from build123d import *

# Parameters (mm, degrees)
BOSS_EXTRUDE1_DEPTH = 5
SKETCH2_W           = 13.8
SKETCH2_H           = 7
BOSS_EXTRUDE2_DEPTH = 5
SKETCH3_W           = 13.8
SKETCH3_H           = 7
BOSS_EXTRUDE3_DEPTH = 5


with BuildPart() as part:
    # Sketch1 → Boss-Extrude1 (new body)
    with BuildSketch(Plane(origin=(0, 0, 0), x_dir=(1, 0, 0), z_dir=(0, 1, 0))):
        Polygon((132.481495242, 9.8), (132.481495242, 4.8), (142.481495242, 4.8), (152.5, 4.8), (152.5, 0), (142.5, 0), (0, 0), (0, 9.8), align=None)
    extrude(amount=BOSS_EXTRUDE1_DEPTH)

    # Sketch2 → Boss-Extrude2 (add)
    with BuildSketch(Plane.ZY.offset(-10)):
        with Locations((-4.9, 3.5)):
            Rectangle(SKETCH2_W, SKETCH2_H)
    extrude(amount=-BOSS_EXTRUDE2_DEPTH)

    # Sketch3 → Boss-Extrude3 (add)
    with BuildSketch(Plane(origin=(30.2, 0, 0), x_dir=(0, 0, -1), z_dir=(1, 0, 0))):
        with Locations((4.9, 3.5)):
            Rectangle(SKETCH3_W, SKETCH3_H)
    extrude(amount=-BOSS_EXTRUDE3_DEPTH)


solid = part.part
For this review, take the finished solid that the model builds, in its own axes (mm). A direction names the side the tool comes from. Coordinates: 2 decimals unless noted, no trailing zeros. Loops run counter-clockwise (first coordinate to the right, second up) from the corner with the lowest first, then second, coordinate; pieces in that order, holes last. Notation, with made-up numbers: (4, 45.25) -> (37, 45.25) arc R21 ccw to (37, 52.25) -> close; hole circle Ø2 at (-37, 55). An arc over 180 degrees is marked (long way). Write each question's results on one line, items separated by ' | '.
Q1. For pin 1 Ø4 at (x, y) = (138, 2) entering from -Z; pin 2 Ø5 at (x, z) = (6.5, -6.5) entering from +Y; pin 3 Ø2.5 at (x, y) = (82.5, 3) entering from -Z, all flat-tipped, find the tip position at first contact; note any pin that passes through.
Taken from the geometry:
pin 1: z = -4.8 | pin 2: y = 5 | pin 3: z = -9.8
Q2. Add section B-B, the plane y = 3.25. State the section outline as (x, z) points, then the cut area to 3 significant figures.
Taken from the geometry:
outline: (0, -9.8) -> (10, -9.8) -> (10, -11.8) -> (15, -11.8) -> (15, -9.8) -> (25.2, -9.8) -> (25.2, -11.8) -> (30.2, -11.8) -> (30.2, -9.8) -> (132.48, -9.8) -> (132.48, -4.8) -> (152.5, -4.8) -> (152.5, 0) -> (30.2, 0) -> (30.2, 2) -> (25.2, 2) -> (25.2, 0) -> (15, 0) -> (15, 2) -> (10, 2) -> (10, 0) -> (0, 0) -> close | area: 1,430 mm²
Q3. Mouldability with a two-part tool opening along X and no side actions: class faces 4 (the flat face through (152.5, 2, -2)), 5 (the flat face through (15, 6, -5)), 6 (the flat face through (12, 3, 2)) as +X half, -X half, draft (parallel to the pull), parting line (faces both ways), or undercut.
Taken from the geometry:
face 4: +X half | face 5: undercut | face 6: draft
Q4. To check wall thickness, follow line 1 along X through (y, z) = (6.75, -6.75); line 2 along Y through (x, z) = (9, -7.25); line 3 along X through (y, z) = (0.75, -6). State the ranges of each line that lie inside material, in increasing order. Write a range as [from, to].
Taken from the geometry:
line 1: [10, 15], [25.2, 30.2] | line 2: [0, 5] | line 3: [0, 132.48]
Q5. Add section A-A, the plane z = -8.5. State the section outline as (x, y) points, then the cut area to 3 significant figures.
Taken from the geometry:
outline: (0, 0) -> (132.48, 0) -> (132.48, 5) -> (30.2, 5) -> (30.2, 7) -> (25.2, 7) -> (25.2, 5) -> (15, 5) -> (15, 7) -> (10, 7) -> (10, 5) -> (0, 5) -> close | area: 682 mm²
Q6. Machinability: for faces 1 (the flat face through (90, 2, 0)), 2 (the flat face through (20, 5, -5)), 3 (the flat face through (5, 2, 0)), which of the approach directions +Z, -Z, +X, -X, +Y, -Y give a long, thin tool a straight path to every point of the face, cutting with its end or side? Answer none if there is none.
Taken from the geometry:
face 1: +Z, +X, +Y, -Y | face 2: +Z, -Z, +Y | face 3: +Z, -X, +Y, -Y
Q7. Add section C-C, the plane x = 142.5. State the section outline as (y, z) points.
Taken from the geometry:
outline: (0, -4.8) -> (5, -4.8) -> (5, 0) -> (0, 0) -> close
Q8. Add section D-D, the plane z = -2.25. State the section outline as (x, y) points.
Taken from the geometry:
outline: (0, 0) -> (152.5, 0) -> (152.5, 5) -> (30.2, 5) -> (30.2, 7) -> (25.2, 7) -> (25.2, 5) -> (15, 5) -> (15, 7) -> (10, 7) -> (10, 5) -> (0, 5) -> close
